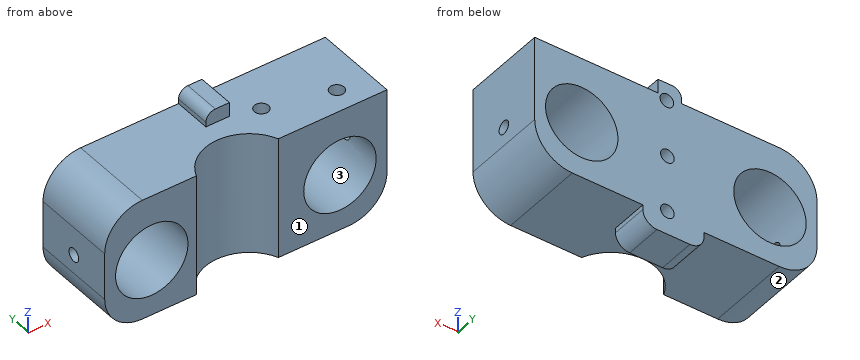
from build123d import *

# Parameters (mm, degrees)
BOX001_W        = 60
BOX001_H        = 18
BOX001_DEPTH    = 26
SKETCH009_R     = 7.7
POCKET007_DEPTH = 21
SKETCH010_R     = 1.4
POCKET008_DEPTH = 5
SKETCH011_R     = 1.5
POCKET009_DEPTH = 5
SKETCH012_R     = 1.4
POCKET010_DEPTH = 5
SKETCH019_W     = 13
SKETCH019_H     = 8
PAD002_DEPTH    = 4
SKETCH020_W     = 5
SKETCH020_H     = 8
PAD003_DEPTH    = 3
SKETCH016_R     = 9.4
POCKET017_DEPTH = 30.001
SKETCH014_R     = 1.45
POCKET018_DEPTH = 6
FILLET003_R     = 2
FILLET004_R     = 3
FILLET005_R     = 8


with BuildPart() as part:
    # Box001 → Box001 (new body)
    with BuildSketch(Plane.XY):
        with Locations((30, 9)):
            Rectangle(BOX001_W, BOX001_H)
    extrude(amount=BOX001_DEPTH)

    # Sketch009 → Pocket007 (cut)
    with BuildSketch(Plane(origin=(0, 18, 0), x_dir=(-1, 0, 0), z_dir=(0, 1, 0))):
        with Locations((-50, 12)):
            Circle(SKETCH009_R)
        with Locations((-10, 12)):
            Circle(SKETCH009_R)
    extrude(amount=-POCKET007_DEPTH, mode=Mode.SUBTRACT)

    # Sketch010 → Pocket008 (cut)
    with BuildSketch(Plane.YZ.offset(60)):
        with Locations((9, 12)):
            Circle(SKETCH010_R)
    extrude(amount=-POCKET008_DEPTH, mode=Mode.SUBTRACT)

    # Sketch011 → Pocket009 (cut)
    with BuildSketch(Plane.XY.offset(26)):
        with Locations((39.5, 8.5)):
            Circle(SKETCH011_R)
        with Locations((53, 5)):
            Circle(SKETCH011_R)
    extrude(amount=-POCKET009_DEPTH, mode=Mode.SUBTRACT)

    # Sketch012 → Pocket010 (cut)
    with BuildSketch(Plane(origin=(0, 0, 0), x_dir=(0, -1, 0), z_dir=(-1, 0, 0))):
        with Locations((-9, 12)):
            Circle(SKETCH012_R)
    extrude(amount=-POCKET010_DEPTH, mode=Mode.SUBTRACT)

    # Sketch019 → Pad002 (new body)
    with BuildSketch(Plane(origin=(0, 0, 0), x_dir=(1, 0, 0), z_dir=(0, 0, -1))):
        with Locations((30.5, -14)):
            Rectangle(SKETCH019_W, SKETCH019_H)
    extrude(amount=PAD002_DEPTH)

    # Sketch020 → Pad003 (new body)
    with BuildSketch(Plane.XY.offset(26)):
        with Locations((31.3, 14)):
            Rectangle(SKETCH020_W, SKETCH020_H)
    extrude(amount=PAD003_DEPTH)

    # Sketch016 → Pocket017 (cut, through all)
    with BuildSketch(Plane.XY.offset(26)):
        with Locations((28.2, -3.5)):
            Circle(SKETCH016_R)
    extrude(amount=-POCKET017_DEPTH, mode=Mode.SUBTRACT)

    # Sketch014 → Pocket018 (cut)
    with BuildSketch(Plane(origin=(0, 18, 0), x_dir=(-1, 0, 0), z_dir=(0, 1, 0))):
        with Locations((-31.8, 13.1)):
            Circle(SKETCH014_R)
        with Locations((-31.8, 1)):
            Circle(SKETCH014_R)
        with Locations((-31.912905, 25.199473)):
            Circle(SKETCH014_R)
    extrude(amount=-POCKET018_DEPTH, mode=Mode.SUBTRACT)

    # Fillet003
    fillet003_edges = [part.edges().sort_by_distance(p)[0] for p in [
        (28.8, 14, 29),
    ]]
    fillet(fillet003_edges, radius=FILLET003_R)

    # Fillet004
    fillet004_edges = [part.edges().sort_by_distance(p)[0] for p in [
        (24, 14, -4),
        (37, 14, -4),
    ]]
    fillet(fillet004_edges, radius=FILLET004_R)

    # Fillet005
    fillet005_edges = [part.edges().sort_by_distance(p)[0] for p in [
        (60, 9, 0),
        (0, 9, 26),
        (0, 9, 0),
    ]]
    fillet(fillet005_edges, radius=FILLET005_R)


solid = part.part
Can you work these out from the model? Positions are in its coordinate system, mm. Face numbers are marked on the shaded views. Give positions to 0.01 mm unless a question says otherwise; leave off trailing zeros. Loops run counter-clockwise (first coordinate to the right, second up) from the corner with the lowest first, then second, coordinate; pieces in that order, holes last. Notation, with made-up numbers: (-2.75, 37.5) - (43.25, 37.5) arc R11 cw to (43.25, 45.5) - close; hole circle Ø1 at (-0.75, 30.25). An arc over 180 degrees is marked (long way). Answer as a JSON object with one key per item and string values.
Q1. Imagine slicing it at B-B on y = 5. Write out the boundary of the cut face in (x, z).
Geometry says:
{"outline": "(0, 8) arc R8 ccw to (8, 0) - (24.19, 0) - (24.19, 26) - (8, 26) arc R8 ccw to (0, 18) - close; (32.21, 0) - (52, 0) arc R8 ccw to (60, 8) - (60, 26) - (54.5, 26) - (54.5, 21) - (51.5, 21) - (51.5, 26) - (32.21, 26) - close; hole circle Ø15.4 at (10, 12); hole circle Ø15.4 at (50, 12)"}
Q2. Imagine slicing it at D-D on z = 15.5. Write out the boundary of the cut face in (x, y), plus the area to 3 significant figures.
Geometry says:
{"outline": "(0, 0) - (3.14, 0) - (3.14, 18) - (0, 18) - close; (16.86, 0) - (19.48, 0) arc R9.4 cw to (36.92, 0) - (43.14, 0) - (43.14, 18) - (16.86, 18) - close; (56.86, 0) - (60, 0) - (60, 18) - (56.86, 18) - close", "area": "512 mm²"}
Q3. If we mould it in two halves opening along X, with no side actions, what happens to the marked faces 1, 2 and 3? For each: pulls with the +X half, pulls with the -X half, needs draft (parallel to the pull), parting line crosses it, or undercut.
Geometry says:
{"face 1": "needs draft", "face 2": "pulls with the -X half", "face 3": "undercut"}
Q4. Imagine slicing it at A-A on x = 50. Write out the boundary of the cut face in (y, z), plus the area to 3 significant figures.
Geometry says:
{"outline": "(0, 0) - (18, 0) - (18, 4.3) - (0, 4.3) - close; (0, 19.7) - (18, 19.7) - (18, 26) - (0, 26) - close", "area": "191 mm²"}
Q5. If I drill on L1, parallel to Z at x = 31.8, y = 16.25; L2, parallel to Y at x = 0.7, z = 12; L3, parallel to X at y = 2.5, z = 18, over which ranges is the centre line in solid material (lowest first)?
Geometry says:
{"L1": "-4 to -0.45, 2.45 to 11.65, 14.55 to 23.75, 26.65 to 29", "L2": "0 to 7.6, 10.4 to 18", "L3": "0 to 5.17, 14.83 to 20.96, 35.44 to 45.17, 54.83 to 60"}
Q6. Imagine slicing it at C-C on z = 22.5. Write out the boundary of the cut face in (x, y).
Geometry says:
{"outline": "(1.39, 0) - (19.48, 0) arc R9.4 cw to (36.92, 0) - (60, 0) - (60, 18) - (1.39, 18) - close; hole circle Ø3 at (39.5, 8.5); hole circle Ø3 at (53, 5)"}
Q7. Will these pins go through, and if not, where does the flat tip stop? P1, Ø1.7, axis at x = 31.8, z = 1, coming from the -Y side; P2, Ø1.5, axis at x = 39, y = 4, coming from the +Z side; P3, Ø2.5, axis at x = 53, y = 5, coming from the +Z side.
Geometry says:
{"P1": "y = 4.78", "P2": "z = 26", "P3": "z = 21"}
